```python
from build123d import *

# Parameters (mm, degrees)
SKETCH1_W           = 50
SKETCH1_H           = 40
BOSS_EXTRUDE1_DEPTH = 20
FILLET1_R           = 3
SKETCH2_W           = 15
SKETCH2_H           = 15
CUT_EXTRUDE1_DEPTH  = 16
SKETCH3_R           = 2.252565919
CUT_EXTRUDE2_DEPTH  = 16
FILLET2_R           = 3
CHAMFER1_SIZE       = 3
CHAMFER1_SIZE2      = 8.242432258
SKETCH4_R           = 4.5
CUT_EXTRUDE3_DEPTH  = 38.749172176
CUT_EXTRUDE4_DEPTH  = 5
SKETCH6_R           = 1.794410379
CUT_EXTRUDE5_DEPTH  = 8
SKETCH7_R           = 0.310906048
BOSS_EXTRUDE2_DEPTH = 4.5


with BuildPart() as part:
    # Sketch1 → Boss-Extrude1 (new body)
    with BuildSketch(Plane(origin=(0, 0, 0), x_dir=(1, 0, 0), z_dir=(0, 1, 0))):
        Rectangle(SKETCH1_W, SKETCH1_H)
    extrude(amount=BOSS_EXTRUDE1_DEPTH)

    # Fillet1
    fillet1_edges = [part.edges().sort_by_distance(p)[0] for p in [
        (25, 10, 20),
        (-25, 10, 20),
        (-25, 10, -20),
        (25, 10, -20),
    ]]
    fillet(fillet1_edges, radius=FILLET1_R)

    # Sketch2 → Cut-Extrude1 (cut)
    with BuildSketch(Plane(origin=(0, 20, 0), x_dir=(1, 0, 0), z_dir=(0, 1, 0))):
        with Locations((-24.121320344, 19.121320344)):
            Rectangle(SKETCH2_W, SKETCH2_H)
        with Locations((24.121320344, 19.121320344)):
            Rectangle(SKETCH2_W, SKETCH2_H)
    extrude(amount=-CUT_EXTRUDE1_DEPTH, mode=Mode.SUBTRACT)

    # Sketch3 → Cut-Extrude2 (cut)
    with BuildSketch(Plane(origin=(0, 4, 0), x_dir=(1, 0, 0), z_dir=(0, 1, 0))):
        with Locations(Location((20.810660172, 15.810660172, 0), (0, 0, 270))):
            Circle(SKETCH3_R)
        with Locations(Location((-20.810660172, 15.810660172, 0), (0, 0, 90))):
            Circle(SKETCH3_R)
    extrude(amount=-CUT_EXTRUDE2_DEPTH, mode=Mode.SUBTRACT)

    # Fillet2
    fillet2_edges = [part.edges().sort_by_distance(p)[0] for p in [
        (-16.621320344, 12, -11.621320344),
        (16.621320344, 12, -11.621320344),
    ]]
    fillet(fillet2_edges, radius=FILLET2_R)

    # Chamfer1
    chamfer1_edges = [part.edges().sort_by_distance(p)[0] for p in [
        (0, 20, -20),
    ]]
    chamfer1_side = [part.faces().sort_by_distance(p)[0] for p in [
        (0, 9.513710794, -20),
    ]]
    chamfer(chamfer1_edges, length=CHAMFER1_SIZE, length2=CHAMFER1_SIZE2, reference=chamfer1_side[0])

    # Sketch4 → Cut-Extrude3 (cut, through all)
    with BuildSketch(Plane(origin=(0, 20, 0), x_dir=(1, 0, 0), z_dir=(0, 1, 0))):
        with Locations(Location((0, -14.79019389, 0), (0, 0, 270))):
            Circle(SKETCH4_R)
    extrude(amount=-CUT_EXTRUDE3_DEPTH, mode=Mode.SUBTRACT)

    # Sketch5 → Cut-Extrude4 (cut)
    with BuildSketch(Plane(origin=(0, 0, -20), x_dir=(-1, 0, 0), z_dir=(0, 0, -1))):
        Polygon((6.87465001, 10.97114015), (-6.87465001, 10.97114015), (-8.382472875, 9.463317285), (-7.628561442, 8.709405853), (7.628561442, 8.709405853), (8.382472875, 9.463317285), align=None)
    extrude(amount=-CUT_EXTRUDE4_DEPTH, mode=Mode.SUBTRACT)

    # Sketch6 → Cut-Extrude5 (cut)
    with BuildSketch(Plane(origin=(0, 0, -20), x_dir=(-1, 0, 0), z_dir=(0, 0, -1))):
        with Locations((13.008166747, 10.460013755)):
            Circle(SKETCH6_R)
        with Locations(Location((-13.008166747, 10.460013755, 0), (0, 0, 180))):
            Circle(SKETCH6_R)
    extrude(amount=-CUT_EXTRUDE5_DEPTH, mode=Mode.SUBTRACT)

    # Sketch7 → Boss-Extrude2 (add)
    with BuildSketch(Plane(origin=(0, 0, -15), x_dir=(-1, 0, 0), z_dir=(0, 0, -1))):
        with Locations(Location((0, 10.357788476, 0), (0, 0, 180))):
            Circle(SKETCH7_R)
        with Locations(Location((1, 10.357788476, 0), (0, 0, 180))):
            Circle(SKETCH7_R)
        with Locations(Location((2, 10.357788476, 0), (0, 0, 180))):
            Circle(SKETCH7_R)
        with Locations(Location((3, 10.357788476, 0), (0, 0, 180))):
            Circle(SKETCH7_R)
        with Locations(Location((4, 10.357788476, 0), (0, 0, 180))):
            Circle(SKETCH7_R)
        with Locations(Location((5, 10.357788476, 0), (0, 0, 180))):
            Circle(SKETCH7_R)
        with Locations(Location((6, 10.357788476, 0), (0, 0, 180))):
            Circle(SKETCH7_R)
        with Locations(Location((1, 9.357788476, 0), (0, 0, 180))):
            Circle(SKETCH7_R)
        with Locations(Location((2, 9.357788476, 0), (0, 0, 180))):
            Circle(SKETCH7_R)
        with Locations(Location((3, 9.357788476, 0), (0, 0, 180))):
            Circle(SKETCH7_R)
        with Locations(Location((4, 9.357788476, 0), (0, 0, 180))):
            Circle(SKETCH7_R)
        with Locations(Location((5, 9.357788476, 0), (0, 0, 180))):
            Circle(SKETCH7_R)
        with Locations(Location((6, 9.357788476, 0), (0, 0, 180))):
            Circle(SKETCH7_R)
        with Locations(Location((0, 9.357788476, 0), (0, 0, 180))):
            Circle(SKETCH7_R)
        with Locations(Location((-6, 9.357788476, 0), (0, 0, 180))):
            Circle(SKETCH7_R)
        with Locations(Location((-5, 9.357788476, 0), (0, 0, 180))):
            Circle(SKETCH7_R)
        with Locations(Location((-4, 9.357788476, 0), (0, 0, 180))):
            Circle(SKETCH7_R)
        with Locations(Location((-3, 9.357788476, 0), (0, 0, 180))):
            Circle(SKETCH7_R)
        with Locations(Location((-2, 9.357788476, 0), (0, 0, 180))):
            Circle(SKETCH7_R)
        with Locations(Location((-1, 9.357788476, 0), (0, 0, 180))):
            Circle(SKETCH7_R)
        with Locations(Location((-6, 10.357788476, 0), (0, 0, 180))):
            Circle(SKETCH7_R)
        with Locations(Location((-5, 10.357788476, 0), (0, 0, 180))):
            Circle(SKETCH7_R)
        with Locations(Location((-4, 10.357788476, 0), (0, 0, 180))):
            Circle(SKETCH7_R)
        with Locations(Location((-3, 10.357788476, 0), (0, 0, 180))):
            Circle(SKETCH7_R)
        with Locations(Location((-2, 10.357788476, 0), (0, 0, 180))):
            Circle(SKETCH7_R)
        with Locations(Location((-1, 10.357788476, 0), (0, 0, 180))):
            Circle(SKETCH7_R)
    extrude(amount=BOSS_EXTRUDE2_DEPTH)


solid = part.part
```
CAD build for the part. Positions are in the model's coordinates, mm. A direction names the side the tool comes from. Coordinates: 2 decimals unless noted, no trailing zeros. Write each loop counter-clockwise with the first axis right and the second up, starting at its lowest first coordinate (ties: lowest second). Pieces come first, ordered by that corner, then holes.
(1) Flat gauge pins, fed straight in: pin 1 (0.7 mm diameter, centred on x = 5, y = 9.5, fed in from -Z); pin 2 (6 mm diameter, centred on x = 22, y = 9.5, fed in from -Z); pin 3 (1.8 mm diameter, centred on x = 13, y = 11, fed in from -Z). Where does each tip first touch, or does it go through?
(2) Cut at B-B, the plane x = 9.5. List the corners of the cut face in (y, z).
(3) Two-plate mould, pull along X, no slides. Class faces 5 (the face through (24.14, 2.03, -19.1)), 6 (the face through (0, 0, 0)), 7 (the face through (0.1, 9.9, -15)): +X half, -X half, draft (parallel to the pull), parting line (faces both ways), or undercut.
(4) Cut at A-A, the plane z = 12. List the corners of the cut face in (x, y), and give its area (3 significant figures).
(5) 3-axis set-ups, long thin cutter, end or side, ignore diameter. For faces 1 (the face through (23, 4, -14)), 2 (the face through (13, 10, -12)), 3 (the face through (-19, 4, -14)), 4 (the face through (-0.26, 18.52, -15.82)): which of +Z, -Z, +X, -X, +Y, -Y reach the whole face in a straight line?
(6) Drill centre lines: probe 1 along X at (y, z) = (9.5, 14.5); probe 2 along X at (y, z) = (11.75, -14.5); probe 3 along Z at (x, y) = (-21, 6). Where is each one in solid material? Low to high.
Geometry says:
1. pin 1: stops at z = -19.5
1. pin 2: stops at z = -11.69
1. pin 3: stops at z = -12
2. outline: (0, -20) - (17, -20) - (20, -11.76) - (20, 20) - (0, 20) - close
3. face 5: +X half
3. face 6: draft
3. face 7: undercut
4. outline: (-25, 0) - (-3.53, 0) - (-3.53, 20) - (-25, 20) - close; (3.53, 0) - (25, 0) - (25, 20) - (3.53, 20) - close
4. area: 859 mm2
5. face 1: -Z, +X, +Y
5. face 2: -Z
5. face 3: -Z, -X, +Y
5. face 4: -Z, +X, -X, +Y
6. probe 1: x = -25 to -4.49, 4.49 to 25
6. probe 2: x = -16.62 to -14.26, -11.76 to 11.76, 14.26 to 16.62
6. probe 3: z = -11.62 to 20
